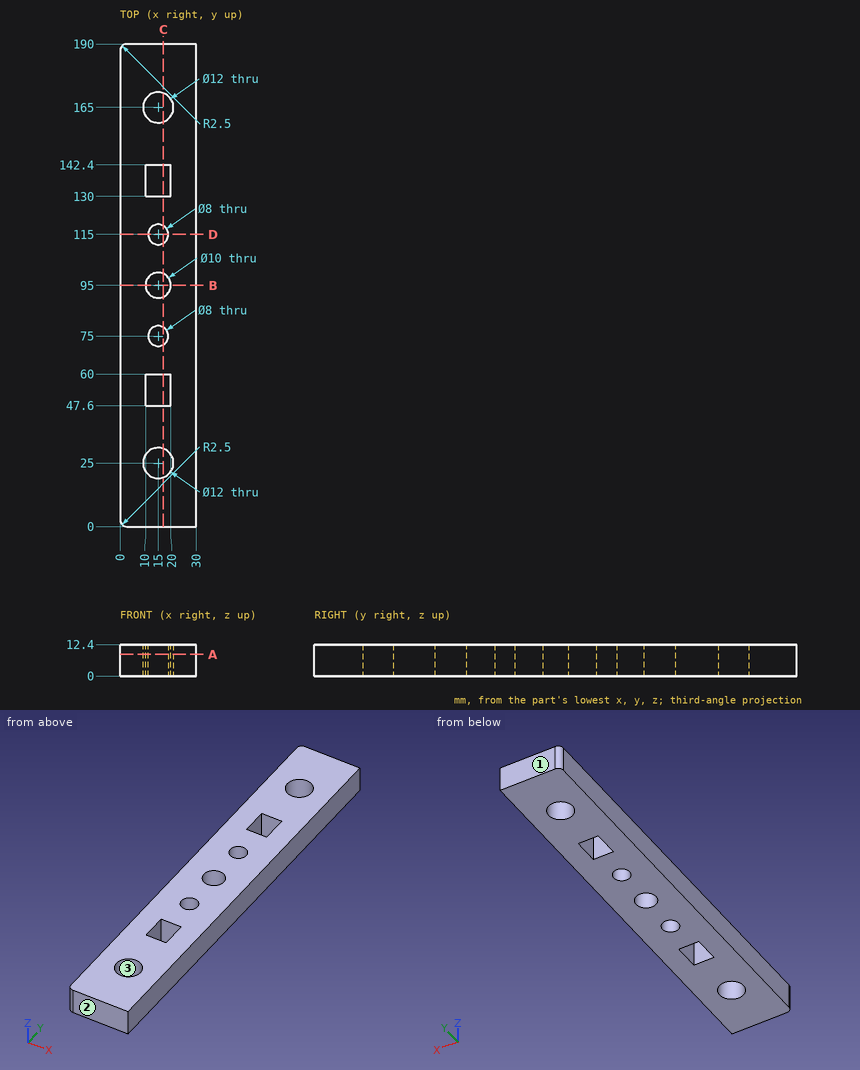
Can you work these out from the drawing? Everything is in mm from the part's minimum corner. Coordinates: 2 decimals unless noted, no trailing zeros. Loops run counter-clockwise (first coordinate to the right, second up) from the corner with the lowest first, then second, coordinate; pieces in that order, holes last.
1. Imagine slicing it at B-B, the plane y = 95. Please give me the cut outline in (x, z), and give its area (3 significant figures).
2. Imagine slicing it at D-D, the plane y = 115. Please give me the cut outline in (x, z), and give its area (3 significant figures).
3. Imagine slicing it at A-A, the plane z = 8.5. Please give me the cut outline in (x, y), and give its area (3 significant figures).
4. For P1, Ø6, axis at x = 15, y = 95, coming from the +Z side; P2, Ø8, axis at x = 15, y = 46.5, coming from the -Z side, each with a flat end and sliding along its axis, tell me the tip position at first contact or that it passes through.
5. I need wall thicknesses on L1, parallel to X at y = 75, z = 8.25; L2, parallel to X at y = 98.5, z = 4.75; L3, parallel to Y at x = 20.5, z = 0.5. Which ranges of each line are inside material? Lowest first, please.
6. If we mould it in two halves opening along Y, with no side actions, what happens to the marked faces 1, 2 and 3? For each: pulls with the +Y half, pulls with the -Y half, needs draft (parallel to the pull), parting line crosses it, or undercut.
7. Imagine slicing it at C-C, the plane x = 17. Count the separate pieces of the cut face and the enclosed holes in it, and give its area (3 significant figures).
Taken from the geometry:
1. outline: (0, 0) - (10, 0) - (10, 12.4) - (0, 12.4) - close; (20, 0) - (30, 0) - (30, 12.4) - (20, 12.4) - close
1. area: 248 mm2
2. outline: (0, 0) - (11, 0) - (11, 12.4) - (0, 12.4) - close; (19, 0) - (30, 0) - (30, 12.4) - (19, 12.4) - close
2. area: 273 mm2
3. outline: (0, 2.5) arc R2.5 ccw to (2.5, 0) - (30, 0) - (30, 190) - (2.5, 190) arc R2.5 ccw to (0, 187.5) - close; hole circle Ø12 at (15, 25); hole circle Ø12 at (15, 165); hole (10, 47.6) - (20, 47.6) - (20, 60) - (10, 60) - close; hole circle Ø10 at (15, 95); hole (10, 130) - (20, 130) - (20, 142.4) - (10, 142.4) - close; hole circle Ø8 at (15, 75); hole circle Ø8 at (15, 115)
3. area: 5,040 mm2
4. P1: passes through
4. P2: stops at z = 0
5. L1: x = 0 to 11, 19 to 30
5. L2: x = 0 to 11.43, 18.57 to 30
5. L3: y = 0 to 22.6, 27.4 to 162.6, 167.4 to 190
6. face 1: pulls with the +Y half
6. face 2: pulls with the -Y half
6. face 3: undercut
7. separate pieces: 8
7. enclosed holes: 0
7. area: 1,480 mm2
